Check sheet for the drawn part. Datum: minimum x, y, z corner. Units: mm. A direction names the side the tool comes from. Round coordinates to 2 decimals unless told otherwise and drop trailing zeros. Write each loop counter-clockwise with the first axis right and the second up, starting at its lowest first coordinate (ties: lowest second). Pieces come first, ordered by that corner, then holes. Notation, with made-up numbers: M 42.25,72.25 L 99.25,72.25 A23 cw 99.25,86.25 Z; hole C 29.25,-25 d8. An arc over 180 degrees is marked long. Answer in a Markdown table with one row per item. Add a question column.
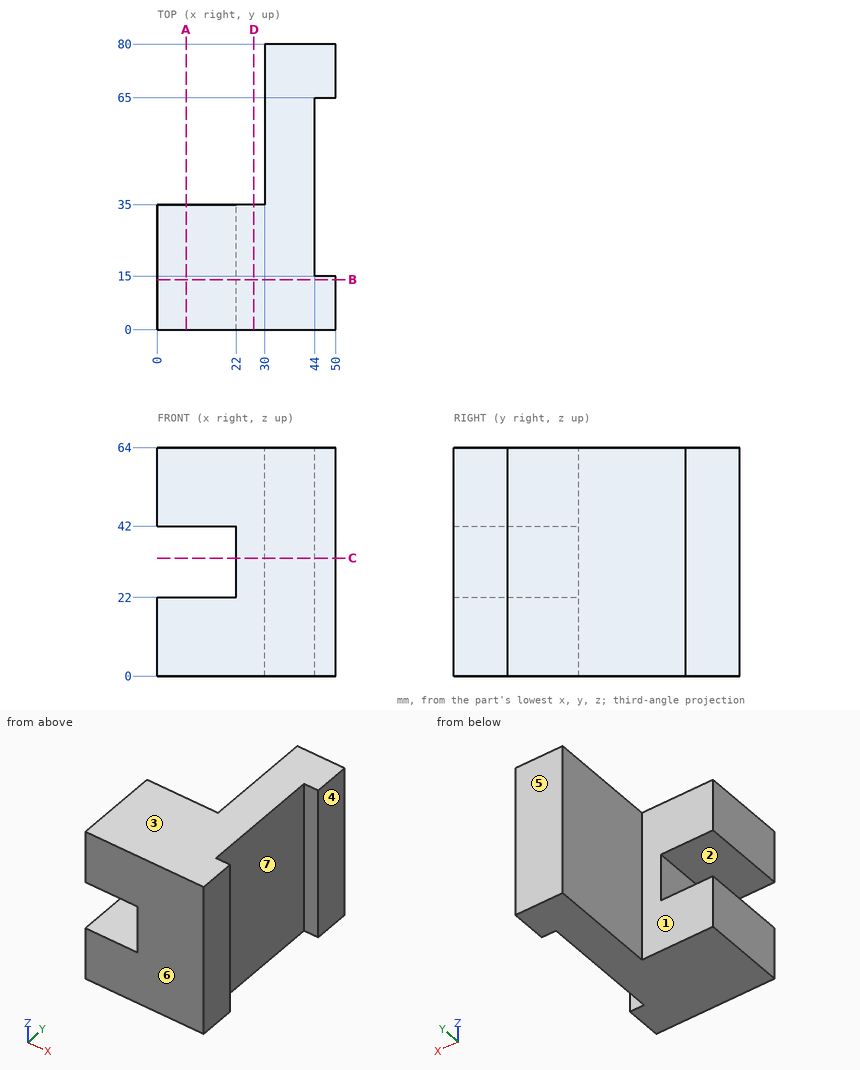
Item 1: Section check C-C, the plane z = 33. Record the boundary of the cut face in (x, y).
Item 2: Section check D-D, the plane x = 27. Record the boundary of the cut face in (y, z).
Item 3: Section check B-B, the plane y = 14. Record the boundary of the cut face in (x, z), and give its area (3 significant figures).
Item 4: Mould release check, pull along Y, two halves, no side actions. Record for the marked faces 4, 5, 6 and 7: +Y half, -Y half, draft (parallel to the pull), parting line (faces both ways), or undercut.
Item 5: Gauge pin test, flat ends, axial feed: pin 1 Ø1.8 at (x, z) = (47.5, 41) entering from -Y; pin 2 Ø13.5 at (y, z) = (64.5, 39.5) entering from -X; pin 3 Ø1.5 at (y, z) = (19.5, 38.5) entering from +X. Record the tip position at first contact, or that the pin passes through.
Item 6: Section check A-A, the plane x = 8. Record the boundary of the cut face in (y, z), and give its area (3 significant figures).
Item 7: Scan lines: probe 1 along Y at (x, z) = (45.5, 34); probe 2 along X at (y, z) = (71, 42.5); probe 3 along Y at (x, z) = (23.5, 14.5). Record each from-to range of solid material in increasing order. Write a range as from..to.
Item 8: Access from +Z, -Z, +X, -X, +Y, -Y to the whole of each face (thin tool, end or side, straight path). Record for the marked faces 1, 2 and 3.
Result sheet:
| question | item | result |
|---|---|---|
| 1 | outline | M 22,0 L 50,0 L 50,15 L 44,15 L 44,65 L 50,65 L 50,80 L 30,80 L 30,35 L 22,35 Z |
| 2 | outline | M 0,0 L 35,0 L 35,64 L 0,64 Z |
| 3 | outline | M 0,0 L 50,0 L 50,64 L 0,64 L 0,42 L 22,42 L 22,22 L 0,22 Z |
| 3 | area | 2,760 mm^2 |
| 4 | face 4 | draft |
| 4 | face 5 | +Y half |
| 4 | face 6 | -Y half |
| 4 | face 7 | undercut |
| 5 | pin 1 | stops at y = 0 |
| 5 | pin 2 | stops at x = 30 |
| 5 | pin 3 | stops at x = 44 |
| 6 | outline | M 0,0 L 35,0 L 35,22 L 0,22 Z; M 0,42 L 35,42 L 35,64 L 0,64 Z |
| 6 | area | 1,540 mm^2 |
| 7 | probe 1 | y = 0..15, 65..80 |
| 7 | probe 2 | x = 30..50 |
| 7 | probe 3 | y = 0..35 |
| 8 | face 1 | +Z, -Z, -X, +Y |
| 8 | face 2 | -X, +Y, -Y |
| 8 | face 3 | +Z, +X, -X, +Y, -Y |
